The listing builds one solid part. Answer for the finished solid, in the listing's coordinates (mm). A direction names the side the tool comes from. Coordinates: 2 decimals unless noted, no trailing zeros. Write each loop counter-clockwise with the first axis right and the second up, starting at its lowest first coordinate (ties: lowest second). Pieces come first, ordered by that corner, then holes.
from build123d import *

# Parameters (mm, degrees)
F0_R          = 6
F0_R_2        = 0.5
F1_DEPTH      = 10
F2_R          = 3
F3_DEPTH      = 40
F4_R          = 1.75
F5_DEPTH      = 10.001
F5_DEPTH_BACK = 10.001
F6_R          = 10
F7_SIZE2      = 3
F7_SIZE       = 2
F7_2_SIZE2    = 3
F7_2_SIZE     = 2


# Not quite as in the source:
# - a pattern or mirror of a feature is missing from the dataset's text; its kind, count and spacing are read off the source's solid


with BuildPart() as f1:
    # F0 (on Front) → F1 (new body)
    with BuildSketch(Plane.XZ):
        with BuildLine():
            Line((71, 5), (8.6602540378, 5))
            ThreePointArc((8.6602540378, 5), (0, 10), (-8.6602540378, 5))
            Line((-8.6602540378, 5), (-72, 5))
            Line((-72, 5), (-72, -5))
            Line((-72, -5), (-8.6602540378, -5))
            ThreePointArc((-8.6602540378, -5), (0, -10), (8.6602540378, -5))
            Line((8.6602540378, -5), (71, -5))
            Line((71, -5), (71, 5))
        make_face()
        Circle(F0_R, mode=Mode.SUBTRACT)
        with Locations((8, 0)):
            Circle(F0_R_2, mode=Mode.SUBTRACT)
    extrude(amount=F1_DEPTH)

    # F2 (on face) → F3 (cut)
    with BuildSketch(Plane(origin=(-72, 0, 0), x_dir=(0, -1, 0), z_dir=(-1, 0, 0))):
        with Locations((5, 0)):
            Circle(F2_R)
    f3 = extrude(amount=-F3_DEPTH, mode=Mode.SUBTRACT)

    # F3_copies: F3 across plane
    add(f3.mirror(Plane(origin=(0, 0, 0), x_dir=(0, 0, 1), z_dir=(1, 0, 0))), mode=Mode.SUBTRACT)

    # F4 (on Top) → F5 (cut, two sides)
    with BuildSketch(Plane.XY) as f5_sk:
        with Locations((0, -5)):
            Circle(F4_R)
    extrude(amount=-F5_DEPTH, mode=Mode.SUBTRACT)
    extrude(f5_sk.sketch, amount=F5_DEPTH_BACK, mode=Mode.SUBTRACT)

    # F6
    f6_edges = [f1.edges().sort_by_distance(p)[0] for p in [
        (-8.660254, -5, 5),
        (8.660254, -5, 5),
        (8.660254, -5, -5),
        (-8.660254, -5, -5),
    ]]
    fillet(f6_edges, radius=F6_R)

    # F7
    f7_edges = [f1.edges().sort_by_distance(p)[0] for p in [
        (-42.614378, -10, 5),
        (-42.614378, -10, -5),
    ]]
    f7_side = f1.faces().sort_by_distance((42.114378, -10, -3.556082))[0]
    chamfer(f7_edges, length=F7_SIZE, length2=F7_SIZE2, reference=f7_side)

    # F7#2
    f7_2_edges = [f1.edges().sort_by_distance(p)[0] for p in [
        (-42.614378, 0, 5),
        (-42.614378, 0, -5),
    ]]
    f7_2_side = f1.faces().sort_by_distance((42.114378, 0, -3.556082))[0]
    chamfer(f7_2_edges, length=F7_2_SIZE, length2=F7_2_SIZE2, reference=f7_2_side)


solid = f1.part
1. Section A-A on x = 57.5 is taken. Give the vertices of the cut face in (y, z), then the cut area to 3 significant figures.
Results found:
outline: (-10, -3) - (-7, -5) - (-3, -5) - (0, -3) - (0, 3) - (-3, 5) - (-7, 5) - (-10, 3) - close; hole circle Ø6 at (-5, 0)
area: 59.7 mm2
2. For a pull along Z with two mould halves and no side action, classify faces 1 (the cylindrical face through (2.769, -4.93, -5.323)), 2 (the flat face through (42, -5, -5)), 3 (the flat face through (-42.2, -1.5, 4)) as pulls with the +Z half, pulls with the -Z half, needs draft (parallel to the pull), parting line crosses it, or undercut.
Results found:
face 1: undercut
face 2: pulls with the -Z half
face 3: pulls with the +Z half
3. Section C-C on y = -5 is taken. State how many separate pieces and enclosed holes the cut face has, then the cut area to 3 significant figures.
Results found:
separate pieces: 2
enclosed holes: 1
area: 946 mm2
4. Find the intervals of material crossed by L1, parallel to Y at x = 0, z = -7.6; L2, parallel to Z at x = -58, y = -5; L3, parallel to X at y = -5, z = 8.2, in increasing order.
Results found:
L1: y = -10 to -6.75, -3.25 to 0
L2: z = -5 to -3, 3 to 5
L3: x = -5.72 to -1.75, 1.75 to 5.72
5. A tool of negligible diameter and unlimited length cuts with its end or side. For faces 4 (the cylindrical face through (51.8, -2.6, -1.8)), 5 (the flat face through (42.5, -1.5, 4)), 6 (the flat face through (42.5, -8.5, 4)), 7 (the flat face through (-32, -5, 0)), 8 (the flat face through (-42.2, -8.5, 4)), from which of +Z, -Z, +X, -X, +Y, -Y can it reach the whole face along a straight path? Write none if from no direction.
Results found:
face 4: +X
face 5: +Z, +X, +Y
face 6: +Z, +X, -Y
face 7: -X
face 8: +Z, -X, -Y
6. Section B-B on x = 0 is taken. Give the vertices of the cut face in (y, z), then the cut area to 3 significant figures.
Results found:
outline: (-10, -8) - (-7, -10) - (-6.75, -10) - (-6.75, -6) - (-10, -6) - close; (-10, 6) - (-6.75, 6) - (-6.75, 10) - (-7, 10) - (-10, 8) - close; (-3.25, -10) - (-3, -10) - (0, -8) - (0, -6) - (-3.25, -6) - close; (-3.25, 6) - (0, 6) - (0, 8) - (-3, 10) - (-3.25, 10) - close
area: 40.0 mm2
7. Flat-ended cylindrical pins translate along their axes: P1, Ø3, axis at x = 22, y = -5, coming from the +Z side; P2, Ø3, axis at x = 31.5, y = -5, coming from the -Z side; P3, Ø5.5, axis at y = -5, z = 0, coming from the -X side. Find the tip coordinate at first contact, or state that the pin passes through.
Results found:
P1: stops at z = 5
P2: stops at z = -5
P3: stops at x = -32
